Source: CAD feature listing. Evaluate the final solid. Frame: model axes, mm. A direction names the side the tool comes from. Coordinates: 2 decimals unless noted, no trailing zeros. Write each loop counter-clockwise with the first axis right and the second up, starting at its lowest first coordinate (ties: lowest second). Pieces come first, ordered by that corner, then holes. Notation, with made-up numbers: (65.5, -3.5) - (117.5, -3.5) arc R14 cw to (117.5, 14.5) - close; hole circle Ø8 at (58, 57.5). An arc over 180 degrees is marked (long way). One line per question, with ' | ' between items. Start each with the question number.
Q1. Access query for faces 4 (the face through (-12.623, -1.51, 109.476)), 5 (the face through (13.28, -0.25, 39.47)). Directions: +Z, -Z, +X, -X, +Y, -Y. A direction counts if a zero-diameter tool reaches every point of the face in a straight line with its end or side. Return the directions, or none.
Q2. Line query: line 1 (Z direction, x = 44.45, y = -1.35) (3 decimals); line 2 (X direction, y = -0.2, z = 2); line 3 (X direction, y = -2, z = 152.4) (3 decimals). Output: solid intervals per line, ascending.
Q3. Contact query for flat-ended pins moving along their axis: P1, Ø1, axis at x = 45, y = -1, coming from the -Z side; P2, Ø1, axis at y = -1.5, z = 80, coming from the +X side; P3, Ø1, axis at x = 7.5, y = -0.5, coming from the -Z side; P4, Ø10, axis at x = 0, z = 152.4, coming from the -Y side. Output: stop coordinate, or through.
Q4. Cut plane B-B, the plane z = 39. Return loops of the section in (x, y).
Q5. Cut plane A-A, the plane y = -1.65. Give the number of separate pieces and of enclosed holes in the cut face, plus the area to 3 significant figures.
Q6. Draft query along X for faces 1 (the face through (13.28, -2.8, 39.47)), 2 (the face through (1.707, -1.51, 66.177)), 3 (the face through (0.192, -0.138, 161.553)). Return one class per face: +X half, -X half, draft (parallel to the pull), parting line (faces both ways), or undercut.
Q7. Cut plane C-C, the plane x = 21. Return loops of the section in (y, z), plus the area to 3 significant figures.
```python
from build123d import *

# Parameters (mm, degrees)
F0_R     = 3.175
F1_DEPTH = 3.048
F2_SIZE  = 0.508
F3_SIZE  = 0.508


with BuildPart() as f1:
    # F0 (on Front) → F1 (new body)
    with BuildSketch(Plane.XZ):
        with BuildLine():
            ThreePointArc((0.340179, -9.518923), (6.854408, -6.613827), (9.525, 0))
            ThreePointArc((9.525, 0), (-0.476848, 9.513056), (-9.477255, -0.9525))
            ThreePointArc((-9.477255, -0.9525), (-6.262383, -7.17692), (0.340179, -9.518923))
        make_face()
        Circle(F0_R, mode=Mode.SUBTRACT)
        with BuildLine():
            ThreePointArc((9.50067, 153.080357), (0, 161.925), (-9.50067, 153.080357))
            ThreePointArc((-9.50067, 153.080357), (-0.340396, 142.881084), (9.525, 152.4))
            ThreePointArc((9.525, 152.4), (9.518916, 152.740396), (9.50067, 153.080357))
        make_face()
        with Locations((0, 152.4)):
            Circle(F0_R, mode=Mode.SUBTRACT)
        with BuildLine():
            ThreePointArc((44.733482, 7.932436), (36.5125, 0), (44.733482, -7.932436))
            ThreePointArc((44.733482, -7.932436), (50.162007, -5.511523), (52.3875, 0))
            ThreePointArc((52.3875, 0), (50.162007, 5.511523), (44.733482, 7.932436))
        make_face()
        with Locations((44.45, 0)):
            Circle(F0_R, mode=Mode.SUBTRACT)
        with BuildLine():
            ThreePointArc((-9.477255, -0.9525), (-0.476848, 9.513056), (9.525, 0))
            ThreePointArc((9.525, 0), (6.854408, -6.613827), (0.340179, -9.518923))
            Line((0.340179, -9.518923), (44.733482, -7.932436))
            ThreePointArc((44.733482, -7.932436), (36.5125, 0), (44.733482, 7.932436))
            Line((44.733482, 7.932436), (18.9676, 8.853234))
            ThreePointArc((18.9676, 8.853234), (13.2612, 11.571359), (11.341187, 17.593382))
            Line((11.341187, 17.593382), (15.795426, 61.9125))
            ThreePointArc((15.795426, 61.9125), (0, 47.625), (-15.795426, 61.9125))
            Line((-15.795426, 61.9125), (-9.477255, -0.9525))
        make_face()
        with BuildLine():
            ThreePointArc((-15.834451, 64.633929), (-15.873368, 63.272376), (-15.795426, 61.9125))
            ThreePointArc((-15.795426, 61.9125), (0, 47.625), (15.795426, 61.9125))
            ThreePointArc((15.795426, 61.9125), (15.855094, 62.705253), (15.875, 63.5))
            ThreePointArc((15.875, 63.5), (15.864859, 64.067327), (15.834451, 64.633929))
            ThreePointArc((15.834451, 64.633929), (0, 79.375), (-15.834451, 64.633929))
        make_face()
        with Locations((0, 63.5)):
            Circle(F0_R, mode=Mode.SUBTRACT)
        with BuildLine():
            Line((-9.50067, 153.080357), (-15.834451, 64.633929))
            ThreePointArc((-15.834451, 64.633929), (0, 79.375), (15.834451, 64.633929))
            Line((15.834451, 64.633929), (9.50067, 153.080357))
            ThreePointArc((9.50067, 153.080357), (9.518916, 152.740396), (9.525, 152.4))
            ThreePointArc((9.525, 152.4), (-0.340396, 142.881084), (-9.50067, 153.080357))
        make_face()
        with Locations((-3.175, 136.5504)):
            Circle(F0_R, mode=Mode.SUBTRACT)
    extrude(amount=F1_DEPTH)

    # F2
    f2_edges = [f1.edges().sort_by_distance(p)[0] for p in [
        (-6.262383, -3.048, -7.17692),
        (22.53683, -3.048, -8.72568),
        (52.3875, -3.048, 0),
        (31.850541, -3.048, 8.392835),
        (13.2612, -3.048, 11.571359),
        (13.568306, -3.048, 39.752941),
        (15.873368, -3.048, 63.272376),
        (12.667561, -3.048, 108.857143),
        (0, -3.048, 161.925),
        (-12.667561, -3.048, 108.857143),
        (-15.873368, -3.048, 63.272376),
        (-12.63634, -3.048, 30.48),
        (-3.175, -3.048, 0),
        (41.275, -3.048, 0),
        (-3.175, -3.048, 63.5),
        (-6.35, -3.048, 136.5504),
        (-3.175, -3.048, 152.4),
    ]]
    chamfer(f2_edges, length=F2_SIZE)

    # F3
    f3_edges = [f1.edges().sort_by_distance(p)[0] for p in [
        (-6.262383, 0, -7.17692),
        (22.53683, 0, -8.72568),
        (52.3875, 0, 0),
        (31.850541, 0, 8.392835),
        (13.2612, 0, 11.571359),
        (13.568306, 0, 39.752941),
        (15.873368, 0, 63.272376),
        (12.667561, 0, 108.857143),
        (0, 0, 161.925),
        (-12.667561, 0, 108.857143),
        (-15.873368, 0, 63.272376),
        (-12.63634, 0, 30.48),
        (-3.175, 0, 0),
        (41.275, 0, 0),
        (-3.175, 0, 63.5),
        (-6.35, 0, 136.5504),
        (-3.175, 0, 152.4),
    ]]
    chamfer(f3_edges, length=F3_SIZE)


solid = f1.part
```
Reply:
1) face 4: +Z, -X, +Y, -Y | face 5: +X, +Y
2) line 1: z = -7.943 to -3.175, 3.175 to 7.943 | line 2: x = -9.46 to -2.85, 2.85 to 41.6, 47.3 to 51.81 | line 3: x = -9.549 to -3.175, 3.175 to 9.549
3) P1: stops at z = -7.94 | P2: stops at x = 14.77 | P3: stops at z = -9.28 | P4: stops at y = -3.05
4) outline: (-13.49, -2.54) - (-12.98, -3.05) - (12.98, -3.05) - (13.49, -2.54) - (13.49, -0.51) - (12.98, 0) - (-12.98, 0) - (-13.49, -0.51) - close
5) separate pieces: 1 | enclosed holes: 5 | area: 4,740 mm^2
6) face 1: +X half | face 2: undercut | face 3: parting line
7) outline: (-3.05, -8.27) - (-2.54, -8.78) - (-0.51, -8.78) - (0, -8.27) - (0, 8.27) - (-0.51, 8.78) - (-2.54, 8.78) - (-3.05, 8.27) - close | area: 53.0 mm^2
